Model file for the job. Use its own axes, mm. Round coordinates to 2 decimals unless told otherwise and drop trailing zeros. Order: outer loops, then holes, each group sorted by start corner. A loop starts at its lowest first (then second) coordinate and runs counter-clockwise, first axis right, second up. Notation, with made-up numbers: M 13.25,79 L 59.25,79 A28 ccw 59.25,99 Z; hole C 54,80.5 d6. An arc over 180 degrees is marked long. Return JSON: item names as keys, results as strings. Group by question number.
Item 1: Slice it at D-D on x = -68. Write the cut outline in (y, z), then the cut area to 3 significant figures.
Item 2: Slice it at B-B on x = 0. Write the cut outline in (y, z).
Item 3: Pull direction Y, two halves, no side cores. Call faces 1 (the face through (-18, 28, 15)), 2 (the face through (-29.97, 1.32, 7.6)), 3 (the face through (-72, -54, 7)): pulls with the +Y half, pulls with the -Y half, needs draft (parallel to the pull), parting line crosses it, or undercut.
Item 4: Slice it at A-A on y = 0. Write the cut outline in (x, z), then the cut area to 3 significant figures.
Item 5: Slice it at C-C on z = 4.5. Write the cut outline in (x, y), then the cut area to 3 significant figures.
Item 6: Probe line 1 along Y through (x, z) = (0.5, 11.25); line 2 along X through (y, z) = (-1, 9.5); line 3 along X through (y, z) = (17, 7.25). List the from-to ranges inside material, lowest first.
from build123d import *

# Parameters (mm, degrees)
SKETCH1_W           = 156
SKETCH1_H           = 120
BOSS_EXTRUDE1_DEPTH = 15
SKETCH2_R           = 30
CUT_EXTRUDE1_DEPTH  = 15
CHAMFER1_SIZE       = 12


with BuildPart() as part:
    # Sketch1 → Boss-Extrude1 (new body)
    with BuildSketch(Plane.XY):
        Rectangle(SKETCH1_W, SKETCH1_H)
    extrude(amount=BOSS_EXTRUDE1_DEPTH)

    # Sketch2 → Cut-Extrude1 (cut)
    with BuildSketch(Plane.XY.offset(15)):
        Circle(SKETCH2_R)
    extrude(amount=-CUT_EXTRUDE1_DEPTH, mode=Mode.SUBTRACT)

    # Chamfer1
    chamfer1_edges = [part.edges().sort_by_distance(p)[0] for p in [
        (78, -60, 7.5),
        (-78, -60, 7.5),
        (-78, 60, 7.5),
        (78, 60, 7.5),
    ]]
    chamfer(chamfer1_edges, length=CHAMFER1_SIZE)


solid = part.part
Output values:
{
 "1": {"outline": "M -58,0 L 58,0 L 58,15 L -58,15 Z", "area": "1,740 mm²"},
 "2": {"outline": "M -60,0 L -30,0 L -30,15 L -60,15 Z; M 30,0 L 60,0 L 60,15 L 30,15 Z"},
 "3": {"face 1": "needs draft", "face 2": "undercut", "face 3": "pulls with the -Y half"},
 "4": {"outline": "M -78,0 L -30,0 L -30,15 L -78,15 Z; M 30,0 L 78,0 L 78,15 L 30,15 Z", "area": "1,440 mm²"},
 "5": {"outline": "M -78,-48 L -66,-60 L 66,-60 L 78,-48 L 78,48 L 66,60 L -66,60 L -78,48 Z; hole C 0,0 d60", "area": "15,600 mm²"},
 "6": {"line 1": "-60 to -30, 30 to 60", "line 2": "-78 to -29.98, 29.98 to 78", "line 3": "-78 to -24.72, 24.72 to 78"}
}
